```python
from build123d import *

# Parameters (mm, degrees)
F0_R          = 12.7
F1_DEPTH      = 17.78
F2_R          = 38.1
F3_DEPTH      = 10.16
F4_R          = 12.954
F5_DEPTH      = 17.781
F5_DEPTH_BACK = 115
F6_W          = 5.08
F6_H          = 30.48
F7_DEPTH      = 38.101
F7_DEPTH_BACK = 38.101
F8_W          = 40.513
F8_H          = 5.08
F9_DEPTH      = 38.101
F9_DEPTH_BACK = 38.101


# Not quite as in the source:
# - an extrude ends at something that could not be found from the text; its depth is read off the source's solid


with BuildPart() as f1:
    # F0 (on Front) → F1 (new body)
    with BuildSketch(Plane.XZ):
        Circle(F0_R)
    extrude(amount=F1_DEPTH)

    # F2 (on Front) → F3 (join)
    with BuildSketch(Plane.XZ):
        Circle(F2_R)
    extrude(amount=F3_DEPTH)

    # F4 (on Front) → F5 (cut, two sides)
    with BuildSketch(Plane.XZ) as f5_sk:
        Circle(F4_R)
    extrude(amount=F5_DEPTH, mode=Mode.SUBTRACT)
    extrude(f5_sk.sketch, amount=-F5_DEPTH_BACK, mode=Mode.SUBTRACT)

    # F6 (on Right) → F7 (cut, two sides)
    with BuildSketch(Plane.YZ) as f7_sk:
        with Locations((-2.54, 0)):
            Rectangle(F6_W, F6_H)
    extrude(amount=F7_DEPTH, mode=Mode.SUBTRACT)
    extrude(f7_sk.sketch, amount=-F7_DEPTH_BACK, mode=Mode.SUBTRACT)

    # F8 (on Top) → F9 (cut, two sides)
    with BuildSketch(Plane.XY) as f9_sk:
        with Locations((-0.7823046945, -2.54)):
            Rectangle(F8_W, F8_H)
    extrude(amount=-F9_DEPTH, mode=Mode.SUBTRACT)
    extrude(f9_sk.sketch, amount=F9_DEPTH_BACK, mode=Mode.SUBTRACT)


solid = f1.part
```
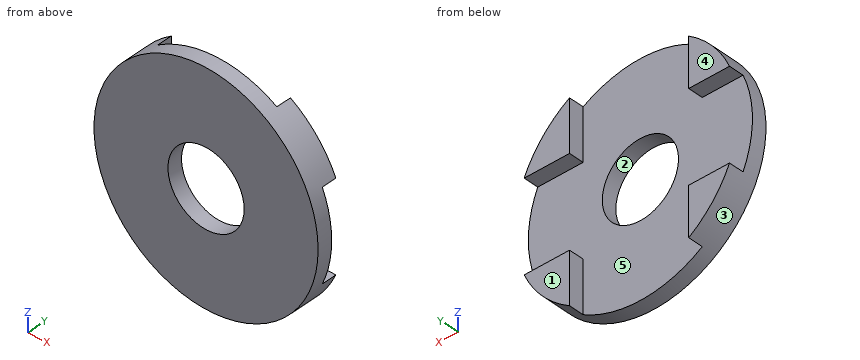
CAD build for the part. Positions are in the model's coordinates, mm. Face numbers are marked on the shaded views. A direction names the side the tool comes from. Round coordinates to 2 decimals unless told otherwise and drop trailing zeros. Write each loop counter-clockwise with the first axis right and the second up, starting at its lowest first coordinate (ties: lowest second). Pieces come first, ordered by that corner, then holes. Notation, with made-up numbers: M 45.25,-19.75 L 67.25,-19.75 A24 cw 67.25,17.25 Z; hole C 6,5.5 d5. An arc over 180 degrees is marked long. One line per question, with ' | ' between items.
1. Probe L1, parallel to Z at x = 0, y = -6.65; L2, parallel to Y at x = 10.5, z = 31. List the from-to ranges inside material, lowest first. Write a range as from..to.
Working result:
L1: -38.1..-12.95, 12.95..38.1 | L2: -10.16..-5.08
2. Cut at D-D on y = -8. Write the cut outline in (x, z), and give its area (3 significant figures).
Working result:
outline: C 0,0 d76.2; hole C 0,0 d25.91 | area: 4,030 mm2
3. Pin check, flat tips, straight feed: pin 1 Ø2.5 at (y, z) = (-2, -27.5) entering from -X; pin 2 Ø1 at (y, z) = (-6.5, 27.5) entering from +X; pin 3 Ø3 at (x, y) = (-8, -5) entering from -Z. Stop position of each tip, or through.
Working result:
pin 1: x = -27.61 | pin 2: x = 26.88 | pin 3: z = -37.54
4. Cut at A-A on x = 0. Write the cut outline in (y, z), and give its area (3 significant figures).
Working result:
outline: M -10.16,-38.1 L -5.08,-38.1 L -5.08,-12.95 L -10.16,-12.95 Z; M -10.16,12.95 L -5.08,12.95 L -5.08,38.1 L -10.16,38.1 Z | area: 255 mm2
5. Which spindle directions (+Z, -Z, +X, -X, +Y, -Y) get a long thin tool onto all of the face, cutting with end or side? Do the marked faces 4 and 5. Say none if no direction does.
Working result:
face 4: +Z, -Z, +X, -X, +Y | face 5: +Y
6. Cut at C-C on z = 0. Write the cut outline in (x, y), and give its area (3 significant figures).
Working result:
outline: M -38.1,-10.16 L -12.95,-10.16 L -12.95,-5.08 L -38.1,-5.08 Z; M 12.95,-10.16 L 38.1,-10.16 L 38.1,-5.08 L 12.95,-5.08 Z | area: 255 mm2
7. Cut at B-B on y = -3.25. Write the cut outline in (x, z), and give its area (3 significant figures).
Working result:
outline: M -34.92,-15.24 A38.1 ccw -21.04,-31.76 L -21.04,-15.24 Z; M -34.92,15.24 L -21.04,15.24 L -21.04,31.76 A38.1 ccw Z; M 19.47,-32.75 A38.1 ccw 34.92,-15.24 L 19.47,-15.24 Z; M 19.47,15.24 L 34.92,15.24 A38.1 ccw 19.47,32.75 Z | area: 602 mm2
8. Mould opens along Z. For the marked faces 1, 2 and 3 say: pulls with the +Z half, pulls with the -Z half, needs draft (parallel to the pull), parting line crosses it, or undercut.
Working result:
face 1: needs draft | face 2: undercut | face 3: parting line crosses it
